```python
from build123d import *

# Parameters (mm, degrees)
EXTRUDE_2_DEPTH     = 9.5
CUT_EXTRUDE_2_REACH = 13.422
SKETCH_4_R          = 2.15


with BuildPart() as part:
    # 草图3 → 凸台-拉伸2 (new body)
    with BuildSketch(Plane.XY):
        with BuildLine():
            Line((-2.7, 0), (2.7, 0))
            ThreePointArc((2.7, 0), (2.912132034, -0.087867966), (3, -0.3))
            Line((3, -0.3), (3, -1))
            Line((3, -1), (4.43, -1))
            ThreePointArc((4.43, -1), (4.65627417, -1.09372583), (4.75, -1.32))
            Line((4.75, -1.32), (4.75, -1.582503942))
            ThreePointArc((4.75, -1.582503942), (4.732643857, -1.695268617), (4.682182017, -1.797595106))
            Line((4.682182017, -1.797595106), (3.089575498, -4.072072931))
            ThreePointArc((3.089575498, -4.072072931), (2.982354469, -4.16610325), (2.843829885, -4.2))
            Line((2.843829885, -4.2), (-2.843829885, -4.2))
            ThreePointArc((-2.843829885, -4.2), (-2.982354469, -4.16610325), (-3.089575498, -4.072072931))
            Line((-3.089575498, -4.072072931), (-4.682182017, -1.797595106))
            ThreePointArc((-4.682182017, -1.797595106), (-4.732643857, -1.695268617), (-4.75, -1.582503942))
            Line((-4.75, -1.582503942), (-4.75, -1.32))
            ThreePointArc((-4.75, -1.32), (-4.65627417, -1.09372583), (-4.43, -1))
            Line((-4.43, -1), (-3, -1))
            Line((-3, -1), (-3, -0.3))
            ThreePointArc((-3, -0.3), (-2.912132034, -0.087867966), (-2.7, 0))
        make_face()
    extrude(amount=EXTRUDE_2_DEPTH)

    # 草图4 → 切除-拉伸2 (cut, up to next)
    with BuildSketch(Plane(origin=(0, 0, 0), x_dir=(1, 0, 0), z_dir=(0, 1, 0)), mode=Mode.PRIVATE) as cut_extrude_2_sk1:
        with Locations(Location((0, -4.75, 0), (0, 0, 180))):
            Circle(SKETCH_4_R)
    cut_extrude_2_tool1 = extrude(cut_extrude_2_sk1.sketch, amount=-CUT_EXTRUDE_2_REACH, mode=Mode.PRIVATE) & part.part
    add(cut_extrude_2_tool1.solids().sort_by_distance((0, 0, 4.75))[0], mode=Mode.SUBTRACT)


solid = part.part
```
Geometry check sheet. Reference: the model listing, model coordinates, mm. A direction names the side the tool comes from. Round coordinates to 2 decimals unless told otherwise and drop trailing zeros. Loops run counter-clockwise (first coordinate to the right, second up) from the corner with the lowest first, then second, coordinate; pieces in that order, holes last. Notation, with made-up numbers: M -12.5,-7 L 41.5,-7 A14 cw 41.5,4 Z; hole C 67,29 d7. An arc over 180 degrees is marked long. Return JSON: item names as keys, results as strings. Group by question number.
(1) Mould release check, pull along X, two halves, no side actions. Record for faces 1 (the face through (-1.2, 0, 2.6)), 2 (the face through (-3.875, -2.951, 4.684)), 3 (the face through (0.28, -2.07, 6.88)): pulls with the +X half, pulls with the -X half, needs draft (parallel to the pull), parting line crosses it, or undercut.
(2) Go/stop test with a flat-tipped pin: pin 1 (1.6 mm diameter, centred on x = -4, z = 6, fed in from +Y). Record where the tip stops, or that it passes through.
(3) Section check C-C, the plane y = -3.25. Enter the section's corners in (x, z).
(4) Scan lines: line 1 along Z through (x, y) = (0, -2.7); line 2 along X through (y, z) = (-0.3, 1.5); line 3 along X through (y, z) = (-1.8, 1). Record each from-to range of solid material in increasing order. Write a range as [from, to].
(5) Section check A-A, the plane x = 0. Enter the section's corners in (y, z).
(6) Set-up check for faces 4 (the face through (-4, -1, 5)), 5 (the face through (4, -1, 5)), 6 (the face through (2, -4.2, 6)): record each of +Z, -Z, +X, -X, +Y, -Y from which the full face is reachable in a straight line by a thin tool's end or side.
Data:
{
 "1": {"face 1": "needs draft", "face 2": "pulls with the -X half", "face 3": "undercut"},
 "2": {"pin 1": "y = -1"},
 "3": {"outline": "M -3.67,0 L 3.67,0 L 3.67,9.5 L -3.67,9.5 Z; hole C 0,4.75 d4.3"},
 "4": {"line 1": "[0, 2.6], [6.9, 9.5]", "line 2": "[-3, 3]", "line 3": "[-4.68, 4.68]"},
 "5": {"outline": "M -4.2,0 L 0,0 L 0,2.6 L -4.2,2.6 Z; M -4.2,6.9 L 0,6.9 L 0,9.5 L -4.2,9.5 Z"},
 "6": {"face 4": "+Z, -Z, -X, +Y", "face 5": "+Z, -Z, +X, +Y", "face 6": "+Z, -Z, +X, -X, -Y"}
}
